Part model, mm, in its own coordinate system. A direction names the side the tool comes from. Round coordinates to 2 decimals unless told otherwise and drop trailing zeros. Write each loop counter-clockwise with the first axis right and the second up, starting at its lowest first coordinate (ties: lowest second). Pieces come first, ordered by that corner, then holes. Notation, with made-up numbers: (42, -24) -> (57, -24) arc R30 cw to (57, 6) -> close; hole circle Ø6 at (-24.75, -4.75). An arc over 180 degrees is marked (long way). Return JSON: item names as keys, results as strings. Group by question number.
(1) Drop flat-ended pins along their axis: pin 1 Ø1.5 at (x, y) = (28, -21.5) entering from +Z; pin 2 Ø12 at (x, y) = (35.5, -17) entering from +Z; pin 3 Ø5 at (x, z) = (10, -11.5) entering from +Y. Give the stop position or say it passes through.
(2) Saw through at C-C (x = 5). List the corners of the cut face in (y, z) (3 decimals).
(3) Drill centre lines: L1, parallel to X at y = -35.5, z = -16.25; L2, parallel to X at y = -15.5, z = -4.5; L3, parallel to Y at x = 47, z = -2. Where is each one in solid material? Low to high. Write a range as from..to.
(4) Mould opens along Z. For faces 1 (the flat face through (25, 0, -3)), 2 (the cylindrical face through (42.37, -35.69, -18.72)), 3 (the cylindrical face through (42.372, -15.169, -6.873)), 4 (the flat face through (25, -5, 0)) say: +Z half, -Z half, draft (parallel to the pull), parting line (faces both ways), or undercut.
(5) Saw through at A-A (y = -4). List the corners of the cut face in (x, z).
(6) Saw through at B-B (x = 13). List the corners of the cut face in (y, z) (3 decimals), plus the area to 3 significant figures.
(7) Saw through at D-D (z = -1.75). List the corners of the cut face in (x, y), plus the area to 3 significant figures.
(8) Tool access for faces 5 (the flat face through (25, -4, -6.35)), 6 (the flat face through (0, -21, -10)): list every direction of +Z, -Z, +X, -X, +Y, -Y with a clear straight run to the whole face (end or side of a thin tool).
Autodesk Inventor part; units mm, degrees
ref_plane "Work Plane1" through (0, -9.525, 0) normal (0, -0.866, -0.5) x (1, 0, 0)
ref_plane "YZ Plane" through (0, 0, 0) normal (1, 0, 0) x (0, 1, 0)
ref_plane "XZ Plane" through (0, 0, 0) normal (0, 1, 0) x (-1, 0, 0)
sketch "Sketch1" plane through (0, 0, 0) normal (1, 0, 0) x (0, 1, 0)
  line L0 (0, 0) -> (-9.525, 0)
  line L1 (-9.525, 0) -> (-9.525, -6.35)
  line L2 (-9.525, -6.35) -> (0, -6.35)
  line L3 (0, -6.35) -> (0, 0)
  dimension "d0" = 9.525
  dimension "d1" = 6.35
extrude "Extrusion1" add sketch "Sketch1" along normal blind 50.8
ref_plane "Work Plane1" through (0, -9.525, 0) normal (0, -0.866, -0.5) x (1, 0, 0)
sketch "Sketch2" plane through (0, -9.525, 0) normal (0, -0.866, -0.5) x (1, 0, 0)
  line L0 (0, 0) -> (50.8, 0)
  line L1 (0, -5.4993) -> (0, -10.2618)
  line L2 (50.8, 0) -> (0, 0)
  line L3 (0, 0) -> (0, -6.35)
  line L4 (0, -6.35) -> (50.8, -6.35)
  line L5 (50.8, -6.35) -> (50.8, 0)
  point P0 (0, -4.7625)
  dimension "d5" = 6.35
extrude "Extrusion2" add sketch "Sketch2" along normal blind 38.1
sketch "Sketch3" plane through (50.8, 0, -6.35) normal (0, 0, -1) x (-1, 0, 0)
  line L0 (50.8, 0) -> (0, 0)
  line L1 (0, -7.8235) -> (0, 0)
  point P0 (3.9118, -3.9118)
  point P1 (46.8882, -3.9118)
  dimension "d8" = 3.9118
  dimension "d9" = 7.8235
  dimension "d10" = 3.9118
  dimension "d11" = 3.9118
  dimension "d12" = 3.9118
hole "Hole1" at (46.8882, -3.9118, -6.35) at (3.9118, -3.9118, -6.35) direction (0, 0, 1) diameter 4.191 end through all
sketch "Sketch4" plane through (50.8, -7.8235, -6.35) normal (0, 0.5, -0.866) x (-1, 0, 0)
  line L0 (0, 0) -> (50.8, 0)
  line L1 (0, 0) -> (0, -36.3985)
  line L2 (50.8, -36.3985) -> (0, -36.3985)
  line L3 (50.8, 0) -> (50.8, -36.3985)
  point P0 (50.8, 9.9504)
  point P1 (44.45, -6.35)
  point P2 (44.45, -30.0485)
  point P3 (6.35, -6.35)
  point P4 (6.35, -30.0485)
  dimension "d20" = 6.35
  dimension "d21" = 6.35
  dimension "d22" = 6.35
  dimension "d23" = 6.35
  dimension "d24" = 6.35
  dimension "d25" = 6.35
  dimension "d26" = 6.35
  dimension "d27" = 6.35
hole "Hole2" at (6.35, -13.3228, -9.525) at (6.35, -33.8463, -21.3743) at (44.45, -13.3228, -9.525) at (44.45, -33.8463, -21.3743) direction (0, -0.5, 0.866) diameter 4.191 end through all
properties part number "PaddleCollection2.1AngleBracket" material "Nylon 6/6"
Computed values:
{
 "1": {"pin 1": "z = -6.48", "pin 2": "z = -0.85", "pin 3": "y = -12.41"},
 "2": {"outline": "(-42.521, -19.05) -> (-39.346, -24.549) -> (-35.234, -22.176) -> (-38.409, -16.676) -> close; (-35.633, -15.074) -> (-32.458, -20.573) -> (-14.711, -10.326) -> (-17.886, -4.827) -> close; (-15.11, -3.224) -> (-11.935, -8.724) -> (-7.824, -6.35) -> (-5.703, -6.35) -> (-5.703, 0) -> (-9.525, 0) -> close; (-2.121, -6.35) -> (0, -6.35) -> (0, 0) -> (-2.121, 0) -> close"},
 "3": {"L1": "0..4.59, 8.11..42.69, 46.21..50.8", "L2": "0..4.35, 8.35..42.45, 46.45..50.8", "L3": "-12.99..-6, -1.82..0"},
 "4": {"face 1": "draft", "face 2": "undercut", "face 3": "undercut", "face 4": "+Z half"},
 "5": {"outline": "(0, -6.35) -> (1.82, -6.35) -> (1.82, 0) -> (0, 0) -> close; (6.01, -6.35) -> (44.79, -6.35) -> (44.79, 0) -> (6.01, 0) -> close; (48.98, -6.35) -> (50.8, -6.35) -> (50.8, 0) -> (48.98, 0) -> close"},
 "6": {"outline": "(-42.521, -19.05) -> (-39.346, -24.549) -> (-7.824, -6.35) -> (0, -6.35) -> (0, 0) -> (-9.525, 0) -> close", "area": "292 mm2"},
 "7": {"outline": "(0, -12.56) -> (50.8, -12.56) -> (50.8, 0) -> (0, 0) -> close; hole circle Ø4.19 at (3.91, -3.91); hole circle Ø4.19 at (46.89, -3.91)", "area": "610 mm2"},
 "8": {"face 5": "-Z, +X, -X, +Y", "face 6": "+Z, -Z, -X, +Y, -Y"}
}
